Design review of the part built by this model. Coordinates are the model's own, in mm. Face numbers are marked on the shaded views. A direction names the side the tool comes from. Round coordinates to 2 decimals unless told otherwise and drop trailing zeros. Loops run counter-clockwise (first coordinate to the right, second up) from the corner with the lowest first, then second, coordinate; pieces in that order, holes last. Notation, with made-up numbers: (-13, -22.5) -> (31, -22.5) arc R20 cw to (31, 11.5) -> close; hole circle Ø1 at (89, 29). An arc over 180 degrees is marked (long way). Answer as CSV lines item,"result". Start each with the question number.
(1) Take a section at A-A, the plane y = 6. Write out the cut boundary in (x, z).
(2) Draft analysis for pull direction X (two halves, no side actions). For the marked faces 1, 2, 3 and 4, state which applies: +X half, -X half, draft (parallel to the pull), parting line (faces both ways), or undercut.
(3) Take a section at B-B, the plane z = -6.75. State how many separate pieces and enclosed holes the cut face has, and give its area (3 significant figures).
(4) For P1, Ø0.8, axis at x = 7.5, z = 1, coming from the -Y side; P2, Ø3.5, axis at y = 5, z = 1.5, coming from the +X side; P3, Ø1.5, axis at y = 10.5, z = 6.5, coming from the -X side; P4, Ø8, axis at x = 1, z = 0.5, coming from the +Y side, all flat-tipped, find the tip position at first contact; note any pin that passes through.
(5) To check wall thickness, follow line 1 (Y direction, x = -7.5, z = -1.25); line 2 (X direction, y = 26, z = 0.25); line 3 (Y direction, x = -1, z = -7). State the ranges of each line that lie inside material, in increasing order. Write a range as from..to.
(6) Take a section at C-C, the plane y = 11. Write out the cut boundary in (x, z), and give its area (3 significant figures).
(7) Machinability: for the marked faces 5, 6 and 7, which of the approach directions +Z, -Z, +X, -X, +Y, -Y give a long, thin tool a straight path to every point of the face, cutting with its end or side? Answer none if there is none.
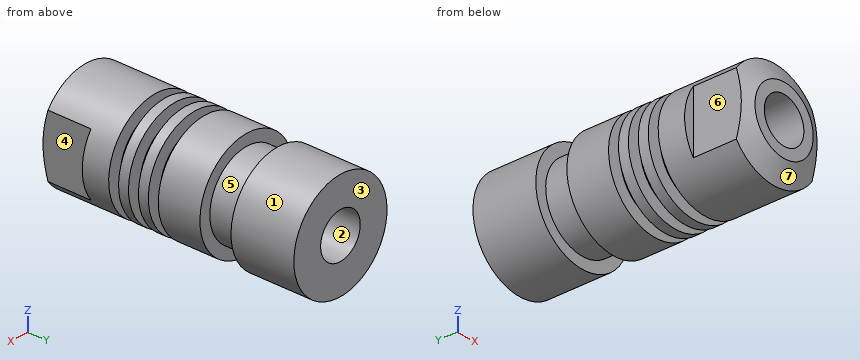
from build123d import *

# Parameters (mm, degrees)
TAGLIO_ESTRUSIONE1_REACH                  = 43.569
TAGLIO_ESTRUSIONE1_END_RADIUS             = 8
SCHIZZO2_W                                = 1.5
SCHIZZO2_H                                = 8
TAGLIO_ESTRUSIONE1_DIRECTION_2_REACH      = 43.569
TAGLIO_ESTRUSIONE1_DIRECTION_2_END_RADIUS = 8
FORO_FILETTATO_M8_1_D                     = 6.8


with BuildPart() as part:
    # Schizzo1 → Rivoluzione1 (revolve)
    with BuildSketch(Plane.XY, mode=Mode.PRIVATE) as rivoluzione1_sk:
        Polygon((0, 0), (-5, 0), (-8, 1.5), (-8, 12), (-6, 12), (-6, 13.5), (-8, 13.5), (-8, 15), (-6, 15), (-6, 16.5), (-8, 16.5), (-8, 18), (-6, 18), (-6, 19.5), (-8, 19.5), (-8, 25.8), (-6.3, 25.8), (-6.3, 30.5), (-8, 30.5), (-8, 40), (0, 40), align=None)
    revolve(rivoluzione1_sk.sketch.rotate(Axis((0, 129.407380346, 0), (0, -1, 0)), 270), axis=Axis((0, 129.407380346, 0), (0, -1, 0)))

    # Taglio-Estrusione1: up to this cylinder (the profile starts inside it)
    taglio_estrusione1_end = Plane(origin=(0, 4, 0), z_dir=(0, 1, 0)) * Cylinder(TAGLIO_ESTRUSIONE1_END_RADIUS, 104.138, mode=Mode.PRIVATE)
    # Schizzo2 → Taglio-Estrusione1 (cut, up to the surface)
    with BuildSketch(Plane.XY, mode=Mode.PRIVATE) as taglio_estrusione1_sk1:
        with Locations((-7.25, 4)):
            Rectangle(SCHIZZO2_W, SCHIZZO2_H)
    taglio_estrusione1_tool1 = extrude(taglio_estrusione1_sk1.sketch, amount=-TAGLIO_ESTRUSIONE1_REACH, mode=Mode.PRIVATE) & taglio_estrusione1_end
    add(taglio_estrusione1_tool1.solids().sort_by_distance((-7.25, 4, 0))[0], mode=Mode.SUBTRACT)
    # Schizzo2 → Taglio-Estrusione1 (cut, up to the surface)
    with BuildSketch(Plane.XY, mode=Mode.PRIVATE) as taglio_estrusione1_sk2:
        with Locations((7.25, 4)):
            Rectangle(SCHIZZO2_W, SCHIZZO2_H)
    taglio_estrusione1_tool2 = extrude(taglio_estrusione1_sk2.sketch, amount=-TAGLIO_ESTRUSIONE1_REACH, mode=Mode.PRIVATE) & taglio_estrusione1_end
    add(taglio_estrusione1_tool2.solids().sort_by_distance((7.25, 4, 0))[0], mode=Mode.SUBTRACT)

    # Taglio-Estrusione1 direction 2: up to this cylinder (the profile starts inside it)
    taglio_estrusione1_direction_2_end = Plane(origin=(0, 4, 0), z_dir=(0, 1, 0)) * Cylinder(TAGLIO_ESTRUSIONE1_DIRECTION_2_END_RADIUS, 104.138, mode=Mode.PRIVATE)
    # Schizzo2 → Taglio-Estrusione1 direction 2 (cut, up to the surface)
    with BuildSketch(Plane.XY, mode=Mode.PRIVATE) as taglio_estrusione1_direction_2_sk1:
        with Locations((-7.25, 4)):
            Rectangle(SCHIZZO2_W, SCHIZZO2_H)
    taglio_estrusione1_direction_2_tool1 = extrude(taglio_estrusione1_direction_2_sk1.sketch, amount=TAGLIO_ESTRUSIONE1_DIRECTION_2_REACH, mode=Mode.PRIVATE) & taglio_estrusione1_direction_2_end
    add(taglio_estrusione1_direction_2_tool1.solids().sort_by_distance((-7.25, 4, 0))[0], mode=Mode.SUBTRACT)
    # Schizzo2 → Taglio-Estrusione1 direction 2 (cut, up to the surface)
    with BuildSketch(Plane.XY, mode=Mode.PRIVATE) as taglio_estrusione1_direction_2_sk2:
        with Locations((7.25, 4)):
            Rectangle(SCHIZZO2_W, SCHIZZO2_H)
    taglio_estrusione1_direction_2_tool2 = extrude(taglio_estrusione1_direction_2_sk2.sketch, amount=TAGLIO_ESTRUSIONE1_DIRECTION_2_REACH, mode=Mode.PRIVATE) & taglio_estrusione1_direction_2_end
    add(taglio_estrusione1_direction_2_tool2.solids().sort_by_distance((7.25, 4, 0))[0], mode=Mode.SUBTRACT)

    # Foro filettato M8-1 (through all)
    with Locations(Plane(origin=(0, 40, 0), x_dir=(1, 0, 0), z_dir=(0, 1, 0))):
        with Locations((0, 0)):
            Hole(FORO_FILETTATO_M8_1_D / 2)


solid = part.part
The answers:
1,outline,"(-6.5, -4.66) arc R8 ccw to (6.5, -4.66) -> (6.5, 4.66) arc R8 ccw to (-6.5, 4.66) -> close; hole circle Ø6.8 at (0, 0)"
2,face 1,"parting line"
2,face 2,"undercut"
2,face 3,"draft"
2,face 4,"+X half"
3,separate pieces,"5"
3,enclosed holes,"0"
3,area,"255 mm²"
4,P1,"y = 8"
4,P2,"x = 6.5"
4,P3,"x = -5.56"
4,P4,"y = 40"
5,line 1,"8..12, 13.5..15, 16.5..18, 19.5..25.8, 30.5..40"
5,line 2,"-6.3..-3.39, 3.39..6.3"
5,line 3,"1.04..12, 13.5..15, 16.5..18, 19.5..25.8, 30.5..40"
6,outline,"circle Ø16 at (0, 0); hole circle Ø6.8 at (0, 0)"
6,area,"165 mm²"
7,face 5,"none"
7,face 6,"+Z, -Z, -X, -Y"
7,face 7,"-Y"
